Check sheet for the drawn part. Datum: minimum x, y, z corner. Units: mm. Give positions to 0.01 mm unless a question says otherwise; leave off trailing zeros. Order: outer loops, then holes, each group sorted by start corner. A loop starts at its lowest first (then second) coordinate and runs counter-clockwise, first axis right, second up. Notation, with made-up numbers: M 48,-3.5 L 68,-3.5 A27 cw 68,17.5 Z; hole C 0,-16.75 d3. An arc over 180 degrees is marked long. Answer in a Markdown table with one row per item. Add a question column.
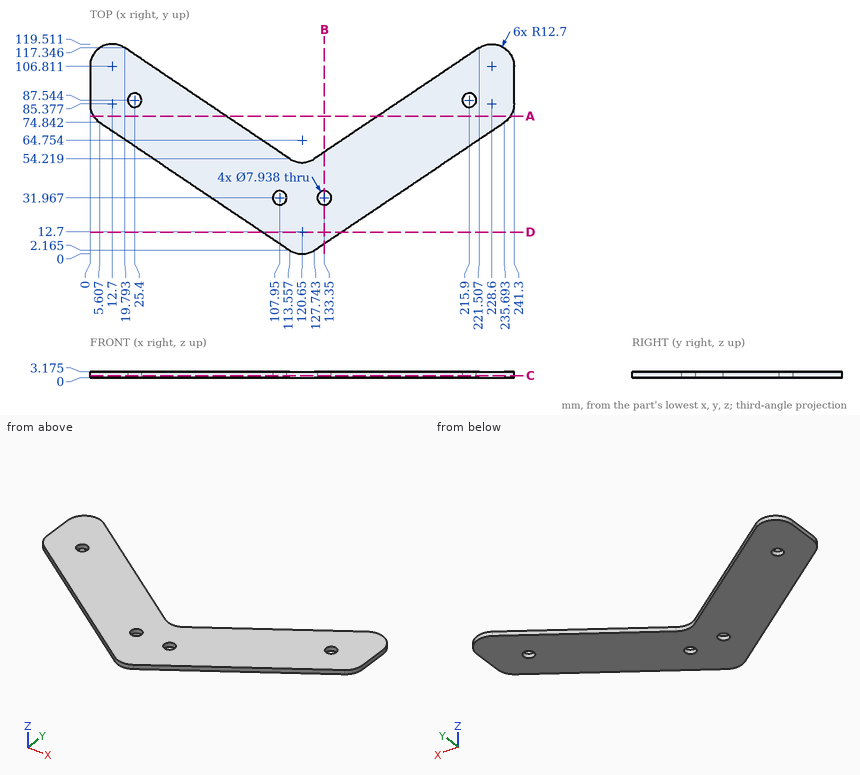
Q1. Go/stop test with flat-tipped pins: pin 1 (7 mm diameter, centred on x = 215.9, y = 87.54, fed in from -Z); pin 2 (1 mm diameter, centred on x = 29, z = 3, fed in from -Y); pin 3 (1.5 mm diameter, centred on x = 131, z = 0.5, fed in from -Y). Record where each tip stops, or that it passes through.
Q2. Cross-section at B-B (x = 133.35). Record the boundary of the cut face in (y, z) (1 decimal), and give its area (3 significant figures).
Q3. Thickness scan on probe 1 along Y at (x, z) = (215.9, 1.4) (1 decimal); probe 2 along Y at (x, z) = (107.95, 0.75) (1 decimal); probe 3 along X at (y, z) = (63.5, 2.15) (1 decimal). Record the ranges inside material, lowest first.
Q4. Cross-section at C-C (z = 1.1). State how many separate pieces and enclosed holes the cut face has, and give its area (3 significant figures).
Q5. Cross-section at D-D (y = 12.5). Record the boundary of the cut face in (x, z) (1 decimal).
Q6. Cross-section at A-A (y = 78.5). Record the boundary of the cut face in (x, z) (1 decimal).
Values follow:
| question | item | result |
|---|---|---|
| 1 | pin 1 | through |
| 1 | pin 2 | y = 58.76 |
| 1 | pin 3 | y = 3.85 |
| 2 | outline | M 5.9,0 L 28,0 L 28,3.2 L 5.9,3.2 Z; M 35.9,0 L 58,0 L 58,3.2 L 35.9,3.2 Z |
| 2 | area | 140 mm² |
| 3 | probe 1 | 61.5 to 83.6, 91.5 to 113.6 |
| 3 | probe 2 | 5.9 to 28, 35.9 to 58 |
| 3 | probe 3 | 22.5 to 99.8, 141.5 to 218.8 |
| 4 | separate pieces | 1 |
| 4 | enclosed holes | 4 |
| 4 | area | 12,100 mm² |
| 5 | outline | M 98.2,0 L 143.1,0 L 143.1,3.2 L 98.2,3.2 Z |
| 6 | outline | M 2,0 L 77.5,0 L 77.5,3.2 L 2,3.2 Z; M 163.8,0 L 239.3,0 L 239.3,3.2 L 163.8,3.2 Z |
